Job drawing, mm, ordinate dimensions from the low corner. One solid piece. A direction names the side the tool comes from. Give positions to 0.01 mm unless a question says otherwise; leave off trailing zeros. Write each loop counter-clockwise with the first axis right and the second up, starting at its lowest first coordinate (ties: lowest second). Pieces come first, ordered by that corner, then holes. Notation, with made-up numbers: M -18,12.25 L 26,12.25 A26 ccw 26,36.25 Z; hole C -7,50 d10. An arc over 180 degrees is marked long. Answer as CSV lines item,"result". Start each with the question number.
Item 1: Band-saw the part on C-C, the plane y = 19. List the corners of the cut face in (x, z).
Item 2: 3-axis set-ups, long thin cutter, end or side, ignore diameter. For the marked faces 1, 2 and 3: which of +Z, -Z, +X, -X, +Y, -Y reach the whole face in a straight line?
Item 3: Pin check, flat tips, straight feed: pin 1 (12 mm diameter, centred on x = 179, y = 153, fed in from -Z); pin 2 (3 mm diameter, centred on x = 88.5, y = 44.5, fed in from +Z). Stop position of each tip, or through.
Item 4: Two-plate mould, pull along Y, no slides. Class the marked faces 4, 5 and 6: +Y half, -Y half, draft (parallel to the pull), parting line (faces both ways), or undercut.
Item 5: Band-saw the part on D-D, the plane x = 82.5. List the corners of the cut face in (y, z).
Item 6: Band-saw the part on B-B, the plane z = 16. List the corners of the cut face in (x, y).
Item 7: Wall check: L1, parallel to Y at x = 132.5, z = 31; L2, parallel to X at y = 83.5, z = 8; L3, parallel to X at y = 96, z = 55.5. Give the ranges that are in metal, low to high. Write a range as from..to.
Item 8: Band-saw the part on A-A, the plane x = 115.5. List the corners of the cut face in (y, z), then the cut area to 3 significant figures.
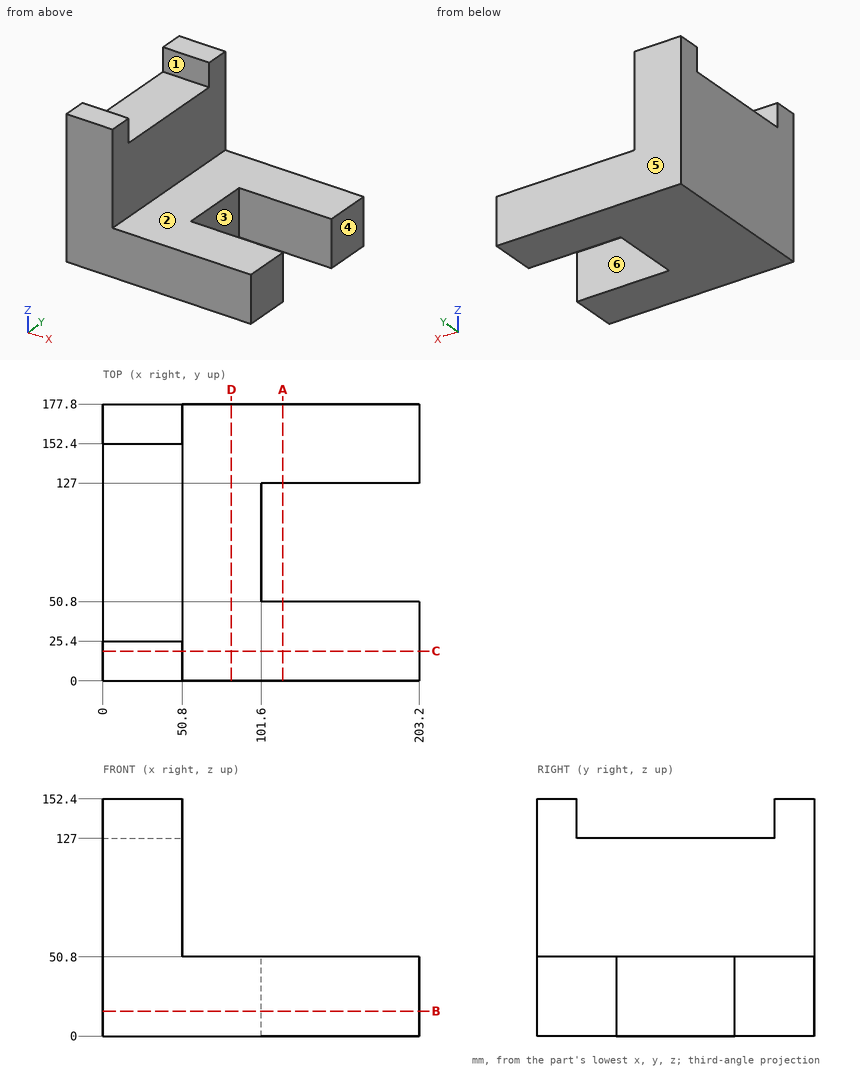
Output:
1,outline,"M 0,0 L 203.2,0 L 203.2,50.8 L 50.8,50.8 L 50.8,152.4 L 0,152.4 Z"
2,face 1,"+Z, +X, -X"
2,face 2,"+Z, +X, +Y, -Y"
2,face 3,"+Z, -Z, +X"
3,pin 1,"z = 0"
3,pin 2,"z = 50.8"
4,face 4,"draft"
4,face 5,"+Y half"
4,face 6,"undercut"
5,outline,"M 0,0 L 177.8,0 L 177.8,50.8 L 0,50.8 Z"
6,outline,"M 0,0 L 203.2,0 L 203.2,50.8 L 101.6,50.8 L 101.6,127 L 203.2,127 L 203.2,177.8 L 0,177.8 Z"
7,L1,"0..50.8, 127..177.8"
7,L2,"0..101.6"
7,L3,"0..50.8"
8,outline,"M 0,0 L 50.8,0 L 50.8,50.8 L 0,50.8 Z; M 127,0 L 177.8,0 L 177.8,50.8 L 127,50.8 Z"
8,area,"5,160 mm²"
